Source: three-view drawing plus pictorial views. Frame: mm from the lowest corner of the part. Give positions to 0.01 mm unless a question says otherwise; leave off trailing zeros. Order: outer loops, then holes, each group sorted by start corner. A loop starts at its lowest first (then second) coordinate and runs counter-clockwise, first axis right, second up.
1) Section B-B, the plane z = 1.1. Give the number of separate pieces and of enclosed holes in the cut face, plus the area to 3 significant figures.
2) Material intervals for line 1 (Y direction, x = 11, z = 1.8); line 2 (X direction, y = 12.5, z = 0.45); line 3 (X direction, y = 5.5, z = 0.45), sorted ascending.
3) Section A-A, the plane x = 71. Return loops of the section in (y, z), plus the area to 3 significant figures.
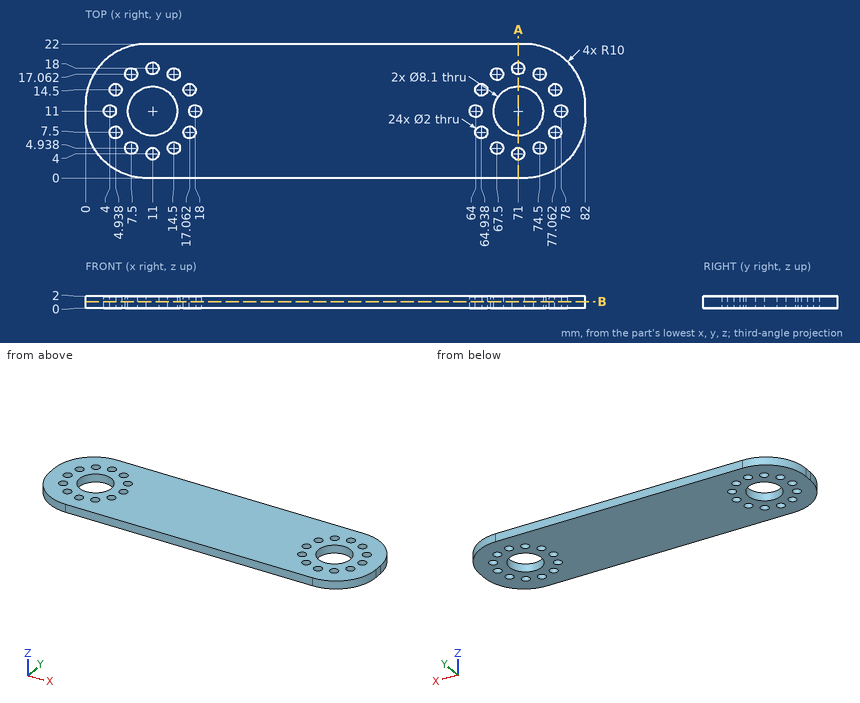
From the geometry:
1. separate pieces: 1
1. enclosed holes: 26
1. area: 1,540 mm2
2. line 1: y = 0 to 3, 5 to 6.95, 15.05 to 17, 19 to 22
2. line 2: x = 0.01 to 7.24, 14.76 to 67.24, 74.76 to 81.99
2. line 3: x = 1.07 to 6.67, 8.33 to 13.67, 15.33 to 66.67, 68.33 to 73.67, 75.33 to 80.93
3. outline: (0, 0) - (3, 0) - (3, 2) - (0, 2) - close; (5, 0) - (6.95, 0) - (6.95, 2) - (5, 2) - close; (15.05, 0) - (17, 0) - (17, 2) - (15.05, 2) - close; (19, 0) - (22, 0) - (22, 2) - (19, 2) - close
3. area: 19.8 mm2
